from build123d import *

# Parameters (mm, degrees)
BOSS_EXTRUDE1_DEPTH = 40
SKETCH2_R           = 4.826
CUT_EXTRUDE2_DEPTH  = 81.20668613
SKETCH6_W           = 40
SKETCH6_H           = 32.7
BOSS_EXTRUDE2_DEPTH = 30
BOSS_EXTRUDE3_START = 91.35
SKETCH7_W           = 60
SKETCH7_H           = 56
BOSS_EXTRUDE3_DEPTH = 20
SKETCH8_W           = 54.5
SKETCH8_H           = 50.5
CUT_EXTRUDE3_DEPTH  = 15
BOSS_EXTRUDE4_DEPTH = 39.65
SKETCH10_W          = 25.001249969
SKETCH10_H          = 3
BOSS_EXTRUDE5_DEPTH = 12
FILLET1_R           = 1.5
FILLET2_R           = 1.5
FILLET3_R           = 1.5


with BuildPart() as part:
    # Sketch1 → Boss-Extrude1 (new body)
    with BuildSketch(Plane(origin=(0, 0, 0), x_dir=(0, 0, -1), z_dir=(1, 0, 0))):
        with BuildLine():
            Line((-10, 0), (-10, 53.5))
            ThreePointArc((-10, 53.5), (-9.560660172, 54.560660172), (-8.5, 55))
            Line((-8.5, 55), (8.5, 55))
            ThreePointArc((8.5, 55), (9.560660172, 54.560660172), (10, 53.5))
            Line((10, 53.5), (10, 35))
            Line((10, 35), (16.35, 35))
            Line((16.35, 35), (16.35, 61.35))
            Line((16.35, 61.35), (-16.35, 61.35))
            Line((-16.35, 61.35), (-16.35, 0))
            Line((-16.35, 0), (-10, 0))
        make_face()
    extrude(amount=BOSS_EXTRUDE1_DEPTH)

    # Sketch2 → Cut-Extrude2 (cut, through all)
    with BuildSketch(Plane.XY.offset(16.35)):
        with Locations((10.25, 20)):
            Circle(SKETCH2_R)
        with Locations(Location((29.75, 20, 0), (0, 0, 270))):
            Circle(SKETCH2_R)
    extrude(amount=-CUT_EXTRUDE2_DEPTH, mode=Mode.SUBTRACT)

    # Sketch6 → Boss-Extrude2 (add)
    with BuildSketch(Plane(origin=(0, 61.35, 0), x_dir=(1, 0, 0), z_dir=(0, 1, 0))):
        with Locations((20, 0)):
            Rectangle(SKETCH6_W, SKETCH6_H)
    extrude(amount=BOSS_EXTRUDE2_DEPTH)

    # Sketch7 → Boss-Extrude3 (add)
    with BuildSketch(Plane(origin=(0, 0, 0), x_dir=(1, 0, 0), z_dir=(0, 1, 0)).offset(BOSS_EXTRUDE3_START)):
        with Locations((20, 0)):
            Rectangle(SKETCH7_W, SKETCH7_H)
    extrude(amount=BOSS_EXTRUDE3_DEPTH)

    # Sketch8 → Cut-Extrude3 (cut)
    with BuildSketch(Plane(origin=(0, 111.35, 0), x_dir=(1, 0, 0), z_dir=(0, 1, 0))):
        with Locations((20, 0)):
            Rectangle(SKETCH8_W, SKETCH8_H)
    extrude(amount=-CUT_EXTRUDE3_DEPTH, mode=Mode.SUBTRACT)

    # Sketch9 → Boss-Extrude4 (add)
    with BuildSketch(Plane(origin=(0, 111.35, 0), x_dir=(1, 0, 0), z_dir=(0, 1, 0))):
        Polygon((2, -25.25), (27, -25), (27, -28), (2, -28), align=None)
    boss_extrude4 = extrude(amount=BOSS_EXTRUDE4_DEPTH)

    # Sketch10 → Boss-Extrude5 (add)
    with BuildSketch(Plane(origin=(3.999900008, 0, 25.230001), x_dir=(0.9999500037496876, 0, -0.00999950003749703), z_dir=(0.00999950003749703, 0, 0.9999500037496877))):
        with Locations((10.500624984, 149.5)):
            Rectangle(SKETCH10_W, SKETCH10_H)
    boss_extrude5 = extrude(amount=-BOSS_EXTRUDE5_DEPTH)

    # Mirror1: Boss-Extrude4, Boss-Extrude5 across plane
    add(boss_extrude4.mirror(Plane.XY))
    add(boss_extrude5.mirror(Plane.XY))

    # Fillet1
    fillet1_edges = [part.edges().sort_by_distance(p)[0] for p in [
        (14.5, 151, -28),
        (14.5, 151, 28),
    ]]
    fillet(fillet1_edges, radius=FILLET1_R)

    # Fillet2
    fillet2_edges = [part.edges().sort_by_distance(p)[0] for p in [
        (0, 45.675, 16.35),
        (0, 63.175, -16.35),
        (40, 63.175, -16.35),
        (40, 45.675, 16.35),
        (50, 101.35, -28),
        (-10, 101.35, -28),
        (-10, 101.35, 28),
        (50, 101.35, 28),
    ]]
    fillet(fillet2_edges, radius=FILLET2_R)

    # Fillet3
    fillet3_edges = [part.edges().sort_by_distance(p)[0] for p in [
        (20, 91.35, 28),
        (20, 91.35, -28),
        (50, 91.35, 0),
        (-10, 91.35, 0),
        (49.560660172, 91.35, 27.560660172),
        (49.560660172, 91.35, -27.560660172),
        (-9.560660172, 91.35, -27.560660172),
        (-9.560660172, 91.35, 27.560660172),
    ]]
    fillet(fillet3_edges, radius=FILLET3_R)


solid = part.part
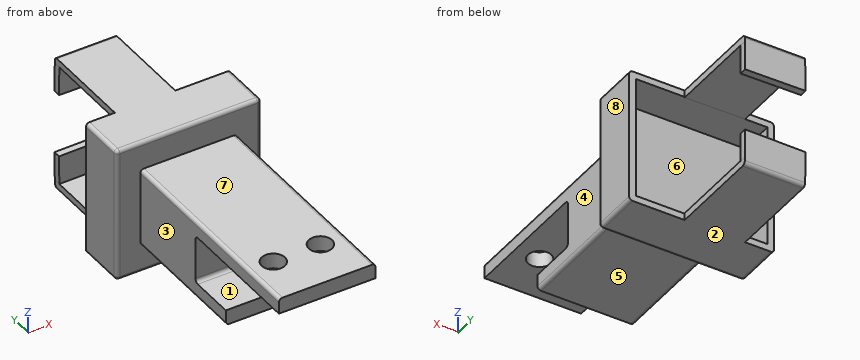
Verification items for the finished model (mm, model axes). Face numbers are marked on the shaded views. A direction names the side the tool comes from. Round coordinates to 2 decimals unless told otherwise and drop trailing zeros. Loops run counter-clockwise (first coordinate to the right, second up) from the corner with the lowest first, then second, coordinate; pieces in that order, holes last. Notation, with made-up numbers: M -32.5,-5 L 24.5,-5 A21 ccw 24.5,15 Z; hole C -5.5,-10 d6. An arc over 180 degrees is marked long. Write each question's results on one line, items separated by ' | '.
1) Access from +Z, -Z, +X, -X, +Y, -Y to the whole of each face (thin tool, end or side, straight path). Record for the marked faces 1, 2, 3, 4 and 5.
Checks:
face 1: +X, -X, -Y | face 2: -Z, +X, -X, +Y, -Y | face 3: +Z, -Z, -X, -Y | face 4: +Z, -Z, +X, -Y | face 5: -Z, +X, -X, -Y
2) Section check C-C on y = 20. Record the boundary of the cut face in (x, z), then the cut area to 3 significant figures.
Checks:
outline: M 0,10 L 5.42,10 L 5.42,16.35 L 1.5,16.35 A1.5 ccw 0,14.85 Z; M 15.08,10 L 24.92,10 L 24.92,16.35 L 15.08,16.35 Z; M 34.58,10 L 40,10 L 40,14.85 A1.5 ccw 38.5,16.35 L 34.58,16.35 Z | area: 130 mm2
3) Section check A-A on y = 121. Record the boundary of the cut face in (x, z).
Checks:
outline: M 2,-28 L 27,-28 L 27,-25 L 2,-25.25 Z; M 2,25.25 L 27,25 L 27,28 L 2,28 Z
4) Scan lines: L1, parallel to Y at x = 10, z = 15; L2, parallel to X at y = 98, z = 19.5; L3, parallel to Y at x = 23, z = -19. Record each from-to range of solid material in increasing order. Write a range as from..to.
Checks:
L1: y = 0..15.18, 24.82..96.35, 148..151 | L2: x = -10..-7.25, 47.25..50 | L3: y = 91.35..96.35, 148..151
5) Section check D-D on z = -6. Record the boundary of the cut face in (x, y).
Checks:
outline: M -10,92.85 A1.5 ccw -8.5,91.35 L 0,91.35 L 0,55 L 40,55 L 40,91.35 L 48.5,91.35 A1.5 ccw 50,92.85 L 50,111.35 L 47.25,111.35 L 47.25,96.35 L -7.25,96.35 L -7.25,111.35 L -10,111.35 Z
6) Gauge pin test, flat ends, axial feed: P1, Ø9.5, axis at x = -4.5, z = -9, coming from the +Y side; P2, Ø18.5, axis at x = 14, z = 0.5, coming from the -Y side; P3, Ø0.8, axis at y = 129.5, z = 26.5, coming from the -X side; P4, Ø15, axis at y = 29, z = -3, coming from the +X side. Record the tip position at first contact, or that the pin passes through.
Checks:
P1: stops at y = 111.35 | P2: stops at y = 54.33 | P3: stops at x = 2 | P4: passes through
7) Section check B-B on x = 29.75. Record the boundary of the cut face in (y, z).
Checks:
outline: M 0,10 L 15.17,10 L 15.17,16.35 L 0,16.35 Z; M 24.83,10 L 53.5,10 A1.5 cw 55,8.5 L 55,-8.5 A1.5 cw 53.5,-10 L 35,-10 L 35,-16.35 L 91.35,-16.35 L 91.35,-26.5 A1.5 ccw 92.85,-28 L 111.35,-28 L 111.35,-25.25 L 96.35,-25.25 L 96.35,25.25 L 111.35,25.25 L 111.35,28 L 92.85,28 A1.5 ccw 91.35,26.5 L 91.35,16.35 L 24.83,16.35 Z
8) Mould release check, pull along X, two halves, no side actions. Record for the marked faces 6, 7 and 8: released by +X, released by -X, zero draft, split by the parting line, or undercut.
Checks:
face 6: undercut | face 7: zero draft | face 8: released by +X
